from build123d import *

# Parameters (mm, degrees)
CUT_EXTRUDE1_DEPTH       = 3
FILLET1_R                = 6
CUT_EXTRUDE2_DEPTH       = 192.342624629
CIRPATTERN2_COUNT        = 8
FILLET1_OF_CIRPATTERN2_R = 6


with BuildPart() as part:
    # Sketch1 → Revolve1 (revolve)
    with BuildSketch(Plane.XY, mode=Mode.PRIVATE) as revolve1_sk:
        with BuildLine():
            Line((116.25, 45), (132, 45))
            Line((132, 45), (132, 38.55))
            Line((132, 38.55), (114, 38.55))
            Line((114, 38.55), (107.202594894, 0))
            Line((107.202594894, 0), (0, 0))
            Line((0, 0), (0, 73.7))
            ThreePointArc((0, 73.7), (59.870177259, 66.418880012), (116.25, 45))
        make_face()
    revolve(revolve1_sk.sketch.rotate(Axis((0, 0, 0), (0, 1, 0)), 90), axis=Axis((0, 0, 0), (0, 1, 0)))

    # Sketch2 → Cut-Extrude1 (cut)
    with BuildSketch(Plane(origin=(0, 45, 0), x_dir=(1, 0, 0), z_dir=(0, 1, 0))):
        with BuildLine():
            Line((130.492133479, 6), (120.18, 6))
            Line((120.18, 6), (120.18, -6))
            Line((120.18, -6), (130.492133479, -6))
            ThreePointArc((130.492133479, -6), (130.63, 0), (130.492133479, 6))
        make_face()
    cut_extrude1 = extrude(amount=-CUT_EXTRUDE1_DEPTH, mode=Mode.SUBTRACT)

    # Fillet1
    fillet1_edges = [part.edges().sort_by_distance(p)[0] for p in [
        (120.18, 43.5, 6),
        (120.18, 43.5, -6),
    ]]
    fillet(fillet1_edges, radius=FILLET1_R - 0.0001)  # a hair under: the kernel refuses the full size

    # Sketch3 → Cut-Extrude2 (cut, through all)
    with BuildSketch(Plane(origin=(0, 42, 0), x_dir=(1, 0, 0), z_dir=(0, 1, 0))):
        with BuildLine():
            Line((125.18, 2.6), (127.18, 2.6))
            ThreePointArc((127.18, 2.6), (129.78, 0), (127.18, -2.6))
            Line((127.18, -2.6), (125.18, -2.6))
            ThreePointArc((125.18, -2.6), (122.58, 0), (125.18, 2.6))
        make_face()
    cut_extrude2 = extrude(amount=-CUT_EXTRUDE2_DEPTH, mode=Mode.SUBTRACT)

    # CirPattern2: Cut-Extrude1, Cut-Extrude2 ×8 about axis
    cirpattern2_axis = Axis((0, 0, 0), (0, 1, 0))
    add([cut_extrude1.rotate(cirpattern2_axis, i * 360 / CIRPATTERN2_COUNT) for i in range(1, CIRPATTERN2_COUNT)], mode=Mode.SUBTRACT)
    add([cut_extrude2.rotate(cirpattern2_axis, i * 360 / CIRPATTERN2_COUNT) for i in range(1, CIRPATTERN2_COUNT)], mode=Mode.SUBTRACT)

    # Fillet1 of CirPattern2
    fillet1_of_cirpattern2_edges = [part.edges().sort_by_distance(p)[0] for p in [
        (89.22273365, 43.5, -80.737452276),
        (80.737452276, 43.5, -89.22273365),
        (6, 43.5, -120.18),
        (-6, 43.5, -120.18),
        (-80.737452276, 43.5, -89.22273365),
        (-89.22273365, 43.5, -80.737452276),
        (-120.18, 43.5, -6),
        (-120.18, 43.5, 6),
        (-89.22273365, 43.5, 80.737452276),
        (-80.737452276, 43.5, 89.22273365),
        (-6, 43.5, 120.18),
        (6, 43.5, 120.18),
        (80.737452276, 43.5, 89.22273365),
        (89.22273365, 43.5, 80.737452276),
    ]]
    fillet(fillet1_of_cirpattern2_edges, radius=FILLET1_OF_CIRPATTERN2_R - 0.0001)  # a hair under: the kernel refuses the full size


solid = part.part
Source: CAD feature listing. Evaluate the final solid. Frame: model axes, mm. A direction names the side the tool comes from. Coordinates: 2 decimals unless noted, no trailing zeros. Loops run counter-clockwise (first coordinate to the right, second up) from the corner with the lowest first, then second, coordinate; pieces in that order, holes last. Notation, with made-up numbers: (44.25, 12) - (67.25, 12) arc R23 ccw to (67.25, 39) - close; hole circle Ø11 at (-21.75, 11). An arc over 180 degrees is marked (long way). Return JSON: item names as keys, results as strings.
Q1. Contact query for flat-ended pins moving along their axis: P1, Ø6, axis at x = -3, y = 49, coming from the +Z side; P2, Ø4, axis at x = -87, y = 10, coming from the +Z side; P3, Ø11.5, axis at x = -127.5, z = 1, coming from the +Y side. Output: stop coordinate, or through.
Results:
{"P1": "z = 114.29", "P2": "z = 68.24", "P3": "y = 45"}
Q2. Section B-B, the plane y = 53. Return loops of the section in (x, z), plus the area to 3 significant figures.
Results:
{"outline": "circle Ø199.12 at (0, 0)", "area": "31,100 mm2"}
Q3. Mould query, pull axis X, two halves, no side actions, for faces 1 (the flat face through (-98, 38.55, 59)), 2 (the cylindrical face through (-39.649, 41.73, -125.904)), 3 (the cylindrical face through (-121.984, 43.479, -4.289)). Classes: released by +X, released by -X, zero draft, split by the parting line, or undercut.
Results:
{"face 1": "zero draft", "face 2": "split by the parting line", "face 3": "undercut"}
Q4. Section A-A, the plane y = 67. Return loops of the section in (x, z).
Results:
{"outline": "circle Ø114.93 at (0, 0)"}
Q5. Access query for faces 4 (the conical face through (95.4, 1.87, -49.62)), 5 (the cylindrical face through (92.31, 43.52, 92.43)). Directions: +Z, -Z, +X, -X, +Y, -Y. A direction counts if a zero-diameter tool reaches every point of the face in a straight line with its end or side. Return the directions, or none.
Results:
{"face 4": "-Y", "face 5": "+Y"}
Q6. Material intervals for line 1 along Y through (x, z) = (37.5, -117.5); line 2 along X through (y, z) = (12, 25); line 3 along Z through (x, y) = (88.5, 3), sorted ascending.
Results:
{"line 1": "38.55 to 45", "line 2": "-106.42 to 106.42", "line 3": "-61.43 to 61.43"}
